from build123d import *

# Parameters (mm, degrees)
BOSS_EXTRUDE1_DEPTH                            = 3
F_3_4_3_4_DIAMETER_HOLE2_D                     = 3.4
CSK_FOR_M3_FLAT_HEAD_MACHINE_SCREW1_AT_2_COUNT = 2
CSK_FOR_M3_FLAT_HEAD_MACHINE_SCREW1_AT_2_PITCH = 28.2
CSK_FOR_M3_FLAT_HEAD_MACHINE_SCREW1_AT_3_COUNT = 2
CSK_FOR_M3_FLAT_HEAD_MACHINE_SCREW1_AT_3_PITCH = 64
CSK_FOR_M3_FLAT_HEAD_MACHINE_SCREW1_AT_4_COUNT = 2
CSK_FOR_M3_FLAT_HEAD_MACHINE_SCREW1_AT_4_PITCH = 69.937400581
CUT_EXTRUDE1_DEPTH                             = 126.193849689
CUT_EXTRUDE1_DEPTH_BACK                        = 10
FILLET1_R                                      = 10
BOSS_EXTRUDE3_START                            = 1.75
SKETCH9_R                                      = 5.5
SKETCH9_R_2                                    = 1.7
BOSS_EXTRUDE3_DEPTH                            = 1.75
SKETCH12_W                                     = 17
SKETCH12_H                                     = 35
SKETCH12_W_2                                   = 19
SKETCH12_H_2                                   = 41.25
SKETCH12_R                                     = 1.7
CUT_EXTRUDE2_DEPTH                             = 114.258081537
CSK_FOR_M3_FLAT_HEAD_MACHINE_SCREW2_AT_2_COUNT = 2
CSK_FOR_M3_FLAT_HEAD_MACHINE_SCREW2_AT_2_PITCH = 79
FILLET2_R                                      = 20
FILLET3_R                                      = 3


with BuildPart() as part:
    # Sketch1 → Boss-Extrude1 (new body)
    with BuildSketch(Plane(origin=(0, 0, 0), x_dir=(1, 0, 0), z_dir=(0, 1, 0))):
        with BuildLine():
            Line((-68.117545464, 56.5), (68.117545464, 56.5))
            ThreePointArc((68.117545464, 56.5), (0, -88.5), (-68.117545464, 56.5))
        make_face()
    extrude(amount=BOSS_EXTRUDE1_DEPTH)

    # Ø3.4 (3.4) Diameter Hole2 (through all)
    with Locations(Plane(origin=(0, 3, 0), x_dir=(1, 0, 0), z_dir=(0, 1, 0))):
        with Locations((69.405322414, -47.216282822), (-83.517603132, -8.443110213), (-69.405322414, -47.216282822), (52.8, 51), (83.517603132, -8.443110213)):
            Hole(F_3_4_3_4_DIAMETER_HOLE2_D / 2)

    # Sketch6 → CSK for M3 Flat Head Machine Screw1 (revolve, cut)
    with BuildSketch(Plane(origin=(32, 3, -46.5), x_dir=(0, 0, 1), z_dir=(1, 0, 0))):
        Polygon((0, 0), (0, 3), (1.7, 3), (1.7, 1.45), (3.15, 0), align=None)
    csk_for_m3_flat_head_machine_screw1 = revolve(axis=Axis((32, 9.35, -46.5), (0, -1, 0)), mode=Mode.SUBTRACT)

    # CSK for M3 Flat Head Machine Screw1 at 2: CSK for M3 Flat Head Machine Screw1 ×2
    with Locations(*[(0, 0, i * CSK_FOR_M3_FLAT_HEAD_MACHINE_SCREW1_AT_2_PITCH) for i in range(1, CSK_FOR_M3_FLAT_HEAD_MACHINE_SCREW1_AT_2_COUNT)]):
        add(csk_for_m3_flat_head_machine_screw1, mode=Mode.SUBTRACT)

    # CSK for M3 Flat Head Machine Screw1 at 3: CSK for M3 Flat Head Machine Screw1 ×2
    with Locations(*[(-i * CSK_FOR_M3_FLAT_HEAD_MACHINE_SCREW1_AT_3_PITCH, 0, 0) for i in range(1, CSK_FOR_M3_FLAT_HEAD_MACHINE_SCREW1_AT_3_COUNT)]):
        add(csk_for_m3_flat_head_machine_screw1, mode=Mode.SUBTRACT)

    # CSK for M3 Flat Head Machine Screw1 at 4: CSK for M3 Flat Head Machine Screw1 ×2
    with Locations(*[Vector(-0.9151040711908488, 0, 0.4032177313684679) * (i * CSK_FOR_M3_FLAT_HEAD_MACHINE_SCREW1_AT_4_PITCH) for i in range(1, CSK_FOR_M3_FLAT_HEAD_MACHINE_SCREW1_AT_4_COUNT)]):
        add(csk_for_m3_flat_head_machine_screw1, mode=Mode.SUBTRACT)

    # Sketch7 → Cut-Extrude1 (cut, two sides: drawn at the far end of the back side and taken through both)
    with BuildSketch(Plane(origin=(0, 3, 0), x_dir=(1, 0, 0), z_dir=(0, 1, 0)).offset(-CUT_EXTRUDE1_DEPTH_BACK)):
        with BuildLine():
            Line((40, -78.944600829), (40, 0.5))
            Line((40, 0.5), (-40, 0.5))
            Line((-40, 0.5), (-40, -78.944600829))
            ThreePointArc((-40, -78.944600829), (0, -88.5), (40, -78.944600829))
        make_face()
    extrude(amount=CUT_EXTRUDE1_DEPTH + CUT_EXTRUDE1_DEPTH_BACK, mode=Mode.SUBTRACT)

    # Fillet1
    fillet1_edges = [part.edges().sort_by_distance(p)[0] for p in [
        (40, 1.5, 78.944600829),
        (-40, 1.5, 78.944600829),
        (40, 1.5, -0.5),
        (-40, 1.5, -0.5),
    ]]
    fillet(fillet1_edges, radius=FILLET1_R)

    # Sketch9 → Boss-Extrude3 (add)
    with BuildSketch(Plane.XZ.offset(BOSS_EXTRUDE3_START)):
        with Locations(Location((52.8, -51, 0), (0, 0, 270))):
            Circle(SKETCH9_R)
        with Locations(Location((52.8, -51, 0), (0, 0, 90))):
            Circle(SKETCH9_R_2, mode=Mode.SUBTRACT)
    extrude(amount=-BOSS_EXTRUDE3_DEPTH)

    # Sketch12 → Cut-Extrude2 (cut, through all)
    with BuildSketch(Plane(origin=(0, 3, 0), x_dir=(1, 0, 0), z_dir=(0, 1, 0))):
        with Locations((-11, 18)):
            Rectangle(SKETCH12_W, SKETCH12_H)
        with Locations((49, 20.875)):
            Rectangle(SKETCH12_W_2, SKETCH12_H_2)
        with Locations(Location((-16.5, 38.5, 0), (0, 0, 270))):
            Circle(SKETCH12_R)
        with Locations(Location((62.5, 38.5, 0), (0, 0, 270))):
            Circle(SKETCH12_R)
    extrude(amount=-CUT_EXTRUDE2_DEPTH, mode=Mode.SUBTRACT)

    # Sketch13 → CSK for M3 Flat Head Machine Screw2 (revolve, cut)
    with BuildSketch(Plane(origin=(62.5, 0, -38.5), x_dir=(0, 0, -1), z_dir=(1, 0, 0))):
        Polygon((0, 0), (0, 3), (1.7, 3), (1.7, 1.45), (3.15, 0), align=None)
    csk_for_m3_flat_head_machine_screw2 = revolve(axis=Axis((62.5, -6.35, -38.5), (0, 1, 0)), mode=Mode.SUBTRACT)

    # CSK for M3 Flat Head Machine Screw2 at 2: CSK for M3 Flat Head Machine Screw2 ×2
    with Locations(*[(-i * CSK_FOR_M3_FLAT_HEAD_MACHINE_SCREW2_AT_2_PITCH, 0, 0) for i in range(1, CSK_FOR_M3_FLAT_HEAD_MACHINE_SCREW2_AT_2_COUNT)]):
        add(csk_for_m3_flat_head_machine_screw2, mode=Mode.SUBTRACT)

    # Fillet2
    fillet2_edges = [part.edges().sort_by_distance(p)[0] for p in [
        (-68.117545464, 1.5, -56.5),
        (68.117545464, 1.5, -56.5),
    ]]
    fillet(fillet2_edges, radius=FILLET2_R)

    # Fillet3
    fillet3_edges = [part.edges().sort_by_distance(p)[0] for p in [
        (-19.5, 1.5, -0.5),
        (-2.5, 1.5, -0.5),
    ]]
    fillet(fillet3_edges, radius=FILLET3_R)


solid = part.part
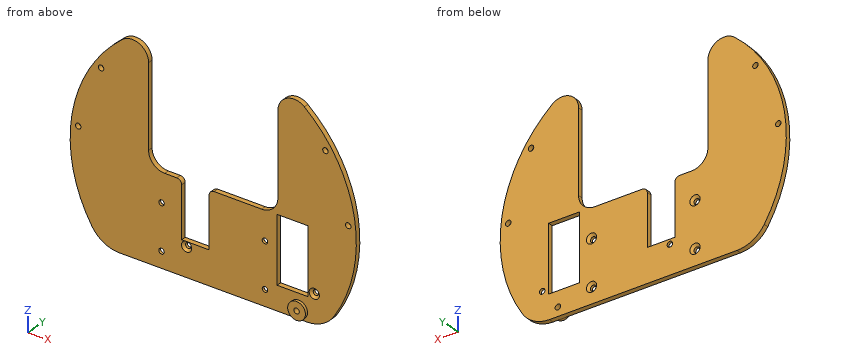
The listing builds one solid part. Answer for the finished solid, in the listing's coordinates (mm). Coordinates: 2 decimals unless noted, no trailing zeros. Order: outer loops, then holes, each group sorted by start corner. A loop starts at its lowest first (then second) coordinate and runs counter-clockwise, first axis right, second up. Notation, with made-up numbers: (11, 36) -> (28, 36) arc R33 cw to (28, 65) -> close; hole circle Ø4 at (86, 36). An arc over 180 degrees is marked (long way). Answer in a Markdown table with one row per item. Add a question column.
Item 1: Find section C-C (x = -46.5). Write down the section's boundary in (y, z), then the cut area to 3 significant figures.
Item 2: Find section B-B (z = 28.5). Write down the section's boundary in (x, y), then the cut area to 3 significant figures.
Item 3: Find the intervals of material crossed by L1, parallel to X at y = 0.8, z = 9.5; L2, parallel to X at y = 0.6, z = -18.3; L3, parallel to X at y = 0.15, z = -48, in increasing order. Write a range as from..to.
Item 4: Each of these flat-tipped pins is pushed along its axis until it touches: P1, Ø2, axis at x = 52.8, z = -51, coming from the +Y side; P2, Ø1.5, axis at y = 1, z = 45, coming from the -X side; P3, Ø1.5, axis at y = 1.5, z = -15, coming from the +X side; P4, Ø2.5, axis at y = 1, z = -27.5, coming from the -X side. Where does it stop, or does it pass through?
Item 5: Find section A-A (z = -26). Write down the section's boundary in (x, y).
Result set:
| question | item | result |
|---|---|---|
| 1 | outline | (0, -56.5) -> (3, -56.5) -> (3, 69.88) -> (0, 69.88) -> close |
| 1 | area | 379 mm² |
| 2 | outline | (-83.79, 0) -> (-40, 0) -> (-40, 3) -> (-83.79, 3) -> close; (40, 0) -> (83.79, 0) -> (83.79, 3) -> (40, 3) -> close |
| 2 | area | 263 mm² |
| 3 | L1 | x = -87.99..-84.85, -82.19..-40, 40..82.19, 84.85..87.99 |
| 3 | L2 | x = -86.59..-33.7, -30.3..-19.5, -2.5..30.3, 33.7..39.5, 58.5..86.59 |
| 3 | L3 | x = -74.33..-32.8, -31.2..31.2, 32.8..74.33 |
| 4 | P1 | passes through |
| 4 | P2 | stops at x = -76.64 |
| 4 | P3 | stops at x = 87.35 |
| 4 | P4 | stops at x = -84.52 |
| 5 | outline | (-84.59, 0) -> (-19.5, 0) -> (-19.5, 3) -> (-84.59, 3) -> close; (-2.5, 0) -> (39.5, 0) -> (39.5, 3) -> (-2.5, 3) -> close; (58.5, 0) -> (84.59, 0) -> (84.59, 3) -> (58.5, 3) -> close |
